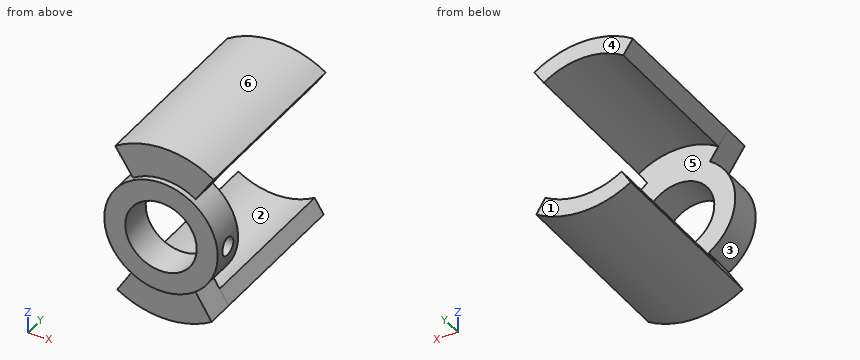
```python
from build123d import *

# Parameters (mm, degrees)
SKETCH1_W                  = 5
SKETCH1_H                  = 3
SKETCH2_R                  = 3.15
CUT_EXTRUDE1_DEPTH         = 8.681145748
M2X0_4_TAPPED_HOLE2_REACH  = 13.576
M2X0_4_TAPPED_HOLE2_BORE_R = 0.8
BOSS_EXTRUDE1_DEPTH        = 13.97
BOSS_EXTRUDE1_2_DEPTH      = 13.97
BOSS_EXTRUDE2_DEPTH        = 2.5


with BuildPart() as part:
    # Sketch1 → Revolve1 (revolve)
    with BuildSketch(Plane.XY, mode=Mode.PRIVATE) as revolve1_sk:
        with Locations((-2.5, -1.5)):
            Rectangle(SKETCH1_W, SKETCH1_H)
    revolve(revolve1_sk.sketch.rotate(Axis((0, 5.888182105, 0), (0, -1, 0)), 270), axis=Axis((0, 5.888182105, 0), (0, -1, 0)))

    # Sketch2 → Cut-Extrude1 (cut, through all)
    with BuildSketch(Plane(origin=(0, 0, 0), x_dir=(1, 0, 0), z_dir=(0, 1, 0))):
        with Locations(Location((0, 0, 0), (0, 0, 270))):
            Circle(SKETCH2_R)
    extrude(amount=-CUT_EXTRUDE1_DEPTH, mode=Mode.SUBTRACT)

    # M2x0.4 Tapped Hole2 bore → M2x0.4 Tapped Hole2 (cut, up to next)
    with BuildSketch(Plane(origin=(5, 0, 0), x_dir=(0, 0, -1), z_dir=(1, 0, 0)), mode=Mode.PRIVATE) as m2x0_4_tapped_hole2_sk1:
        with Locations((0, -1.5)):
            Circle(M2X0_4_TAPPED_HOLE2_BORE_R)
    m2x0_4_tapped_hole2_tool1 = extrude(m2x0_4_tapped_hole2_sk1.sketch, amount=-M2X0_4_TAPPED_HOLE2_REACH, mode=Mode.PRIVATE) & part.part
    add(m2x0_4_tapped_hole2_tool1.solids().sort_by_distance((5, -1.5, 0))[0], mode=Mode.SUBTRACT)



with BuildPart() as body_2:
    # Sketch9 → Boss-Extrude1 (new body)
    with BuildSketch(Plane(origin=(0, 0, 0), x_dir=(1, 0, 0), z_dir=(0, 1, 0))):
        with BuildLine():
            Line((-3.366324533, 5.384269602), (-4.161519304, 6.656144311))
            ThreePointArc((-4.161519304, 6.656144311), (0, 7.85), (4.161519304, 6.656144311))
            Line((4.161519304, 6.656144311), (3.366324533, 5.384269602))
            ThreePointArc((3.366324533, 5.384269602), (0, 6.35), (-3.366324533, 5.384269602))
        make_face()
    extrude(amount=BOSS_EXTRUDE1_DEPTH)


with BuildPart() as body_3:
    # Sketch9 → Boss-Extrude1 2 (new body)
    with BuildSketch(Plane(origin=(0, 0, 0), x_dir=(1, 0, 0), z_dir=(0, 1, 0))):
        with BuildLine():
            Line((3.509629139, -5.291975369), (4.338675392, -6.542048291))
            ThreePointArc((4.338675392, -6.542048291), (0, -7.85), (-4.338675392, -6.542048291))
            Line((-4.338675392, -6.542048291), (-3.509629139, -5.291975369))
            ThreePointArc((-3.509629139, -5.291975369), (0, -6.35), (3.509629139, -5.291975369))
        make_face()
    extrude(amount=BOSS_EXTRUDE1_2_DEPTH)


with BuildPart() as part_1:
    add(part.part)

    add(body_2.part)  # Boss-Extrude2 merges body 2

    add(body_3.part)  # Boss-Extrude2 merges body 3
    # Sketch11 → Boss-Extrude2 (add)
    with BuildSketch(Plane.XZ):
        with BuildLine():
            Line((4.161519304, -6.656144311), (2.650649238, -4.239582363))
            ThreePointArc((2.650649238, -4.239582363), (0, -5), (-2.650649238, -4.239582363))
            Line((-2.650649238, -4.239582363), (-4.161519304, -6.656144311))
            ThreePointArc((-4.161519304, -6.656144311), (0, -7.85), (4.161519304, -6.656144311))
        make_face()
        with BuildLine():
            Line((-4.338675392, 6.542048291), (-2.763487511, 4.166909739))
            ThreePointArc((-2.763487511, 4.166909739), (0, 5), (2.763487511, 4.166909739))
            Line((2.763487511, 4.166909739), (4.338675392, 6.542048291))
            ThreePointArc((4.338675392, 6.542048291), (0, 7.85), (-4.338675392, 6.542048291))
        make_face()
    extrude(amount=BOSS_EXTRUDE2_DEPTH)


solid = part_1.part
```
Design review of the part built by this model. Coordinates are the model's own, in mm. Face numbers are marked on the shaded views. A direction names the side the tool comes from. Coordinates: 2 decimals unless noted, no trailing zeros. Order: outer loops, then holes, each group sorted by start corner. A loop starts at its lowest first (then second) coordinate and runs counter-clockwise, first axis right, second up.
1) Take a section at C-C, the plane x = -1.25. Give the boundary of the cut face in (y, z), and give its area (3 significant figures).
2) Wall thickness on line 1 along Y through (x, z) = (3.8, 0); line 2 along Z through (x, y) = (3.7, -1.5); line 3 along X through (y, z) = (-0.65, 0): over which ranges is each line inside the solid? List them lowest first.
3) Take a section at B-B, the plane y = 3.25. Give the boundary of the cut face in (x, z), and give its area (3 significant figures).
4) Take a section at A-A, the plane z = 0. Give the boundary of the cut face in (x, y).
5) For the marked faces 1 and 2, list the 3-axis set-ups (+Z, -Z, +X, -X, +Y, -Y) from which the entire face can be reached by the end or side of a thin tool; tool diameter is ignored.
6) Take a section at D-D, the plane z = -2.25. Give the boundary of the cut face in (x, y), and give its area (3 significant figures).
7) Mouldability with a two-part tool opening along Z and no side actions: class the marked faces 3, 4, 5 and 6 as +Z half, -Z half, draft (parallel to the pull), parting line (faces both ways), or undercut.
8) Clearance check with flat-ended pins moving along their axes: pin 1 (6 mm diameter, centred on y = 4, z = -0.5, fed in from +X); pin 2 (1 mm diameter, centred on x = 1, y = 2.5, fed in from -Z); pin 3 (2 mm diameter, centred on x = -4, z = -0.5, fed in from +Y); pin 4 (6 mm diameter, centred on y = -0.5, z = -4.5, fed in from -X). State where each tip first meets the part, or that it passes through.
Returned:
1. outline: (-3, -4.84) - (-2.5, -4.84) - (-2.5, -7.75) - (13.97, -7.75) - (13.97, -6.23) - (0, -6.23) - (0, -2.89) - (-3, -2.89) - close; (-3, 2.89) - (0, 2.89) - (0, 6.23) - (13.97, 6.23) - (13.97, 7.75) - (-2.5, 7.75) - (-2.5, 4.84) - (-3, 4.84) - close
1. area: 68.8 mm2
2. line 1: y = -3 to -2.3, -0.7 to 0
2. line 2: z = -6.92 to -5.92, -3.36 to -0.8, 0.8 to 3.36, 5.58 to 6.92
2. line 3: x = -5 to -3.15, 3.15 to 5
3. outline: (-4.34, 6.54) - (-3.51, 5.29) arc R6.35 cw to (3.51, 5.29) - (4.34, 6.54) arc R7.85 ccw to start; (-4.16, -6.66) arc R7.85 ccw to (4.16, -6.66) - (3.37, -5.38) arc R6.35 cw to (-3.37, -5.38) - close
3. area: 24.4 mm2
4. outline: (-5, -3) - (-3.15, -3) - (-3.15, 0) - (-5, 0) - close; (3.15, -3) - (5, -3) - (5, -2.3) - (3.15, -2.3) - close; (3.15, -0.7) - (5, -0.7) - (5, 0) - (3.15, 0) - close
5. face 1: +Z, -Z, +X, -X, +Y
5. face 2: +Y
6. outline: (-4.47, -3) - (-2.2, -3) - (-2.2, 0) - (-4.47, 0) - close; (2.2, -3) - (4.47, -3) - (4.47, 0) - (2.2, 0) - close
6. area: 13.6 mm2
7. face 3: undercut
7. face 4: draft
7. face 5: undercut
7. face 6: +Z half
8. pin 1: passes through
8. pin 2: stops at z = -7.83
8. pin 3: stops at y = 0
8. pin 4: stops at x = -4.77
